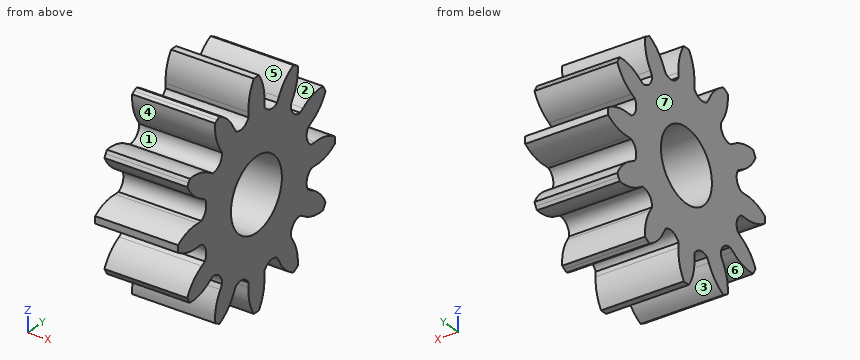
Autodesk Inventor part; units mm, degrees
ref_plane "Work Plane2" through (2.8575, 0, 0) normal (1, 0, 0) x (0, 0, -1)
ref_plane "YZ Plane" through (0, 0, 0) normal (1, 0, 0) x (0, 1, 0)
ref_plane "XZ Plane" through (0, 0, 0) normal (0, 1, 0) x (-1, 0, 0)
ref_plane "Work Plane2" through (2.8575, 0, 0) normal (1, 0, 0) x (0, 0, -1)
sketch "Sketch6" plane through (2.8575, 0, 0) normal (1, 0, 0) x (0, 0, -1)
  line L0 (0.7654, -5.6784) -> (0.7654, -5.022)
  line L1 (-0.7638, -5.6784) -> (-0.7638, -5.0222)
  arc A0 (5.6006, 2.3498) -> (5.5837, 2.3418) centre (6.3532, 0.7382) ccw
  arc A1 (-0.7638, -5.0222) -> (0.7654, -5.022) centre (0, 0) ccw
  line L2 (0.0008, -7.62) -> (-0.2439, -7.62)
  line L3 (0.0008, -7.62) -> (0.2479, -7.62)
  arc A2 (0.2479, -7.62) -> (0.7654, -5.6784) centre (-2.309, -5.8988) ccw
  arc A3 (-0.7638, -5.6784) -> (-0.2439, -7.62) centre (2.2185, -5.9201) ccw
  arc A4 (3.5877, -3.5965) -> (3.5976, -3.5866) centre (0, 0) ccw
  line L4 (3.502, -4.5349) -> (3.1738, -3.9665)
  line L5 (2.1777, -5.2996) -> (1.8496, -4.7313)
  arc A5 (1.8496, -4.7313) -> (3.1738, -3.9665) centre (0, 0) ccw
  line L6 (3.8107, -6.5987) -> (3.5988, -6.721)
  line L7 (3.8107, -6.5987) -> (4.0247, -6.4752)
  arc A6 (4.0247, -6.4752) -> (3.502, -4.5349) centre (0.9498, -6.263) ccw
  arc A7 (2.1777, -5.2996) -> (3.5988, -6.721) centre (4.8813, -4.0177) ccw
  line L8 (5.3003, -2.1764) -> (4.7319, -1.8482)
  line L9 (4.5358, -3.5007) -> (3.9675, -3.1726)
  arc A8 (3.9675, -3.1726) -> (4.7319, -1.8482) centre (0, 0) ccw
  line L10 (6.5995, -3.8093) -> (6.4772, -4.0212)
  line L11 (6.5995, -3.8093) -> (6.7231, -3.5953)
  arc A9 (6.7231, -3.5953) -> (5.3003, -2.1764) centre (3.954, -4.949) ccw
  arc A10 (4.5358, -3.5007) -> (6.4772, -4.0212) centre (6.2362, -1.0388) ccw
  line L12 (5.6784, 0.7654) -> (5.022, 0.7654)
  line L13 (5.6784, -0.7638) -> (5.0222, -0.7638)
  arc A11 (5.0222, -0.7638) -> (5.022, 0.7654) centre (0, 0) ccw
  line L14 (7.62, 0.0008) -> (7.62, -0.2439)
  line L15 (7.62, 0.0008) -> (7.62, 0.2479)
  arc A12 (7.62, 0.2479) -> (5.6784, 0.7654) centre (5.8988, -2.309) ccw
  arc A13 (5.6784, -0.7638) -> (7.62, -0.2439) centre (5.9201, 2.2185) ccw
  line L16 (4.5349, 3.502) -> (3.9665, 3.1738)
  line L17 (5.2996, 2.1777) -> (4.7313, 1.8496)
  arc A14 (4.7313, 1.8496) -> (3.9665, 3.1738) centre (0, 0) ccw
  line L18 (6.5987, 3.8107) -> (6.721, 3.5988)
  line L19 (6.5987, 3.8107) -> (6.4752, 4.0247)
  arc A15 (6.4752, 4.0247) -> (4.5349, 3.502) centre (6.263, 0.9498) ccw
  arc A16 (5.2996, 2.1777) -> (6.721, 3.5988) centre (4.0177, 4.8813) ccw
  line L20 (2.1764, 5.3003) -> (1.8482, 4.7319)
  line L21 (3.5007, 4.5358) -> (3.1726, 3.9675)
  arc A17 (3.1726, 3.9675) -> (1.8482, 4.7319) centre (0, 0) ccw
  line L22 (3.8093, 6.5995) -> (4.0212, 6.4772)
  line L23 (3.8093, 6.5995) -> (3.5953, 6.7231)
  arc A18 (3.5953, 6.7231) -> (2.1764, 5.3003) centre (4.949, 3.954) ccw
  arc A19 (3.5007, 4.5358) -> (4.0212, 6.4772) centre (1.0388, 6.2362) ccw
  line L24 (-0.7654, 5.6784) -> (-0.7654, 5.022)
  line L25 (0.7638, 5.6784) -> (0.7638, 5.0222)
  arc A20 (0.7638, 5.0222) -> (-0.7654, 5.022) centre (0, 0) ccw
  line L26 (-0.0008, 7.62) -> (0.2439, 7.62)
  line L27 (-0.0008, 7.62) -> (-0.2479, 7.62)
  arc A21 (-0.2479, 7.62) -> (-0.7654, 5.6784) centre (2.309, 5.8988) ccw
  arc A22 (0.7638, 5.6784) -> (0.2439, 7.62) centre (-2.2185, 5.9201) ccw
  line L28 (-3.502, 4.5349) -> (-3.1738, 3.9665)
  line L29 (-2.1777, 5.2996) -> (-1.8496, 4.7313)
  arc A23 (-1.8496, 4.7313) -> (-3.1738, 3.9665) centre (0, 0) ccw
  line L30 (-3.8107, 6.5987) -> (-3.5988, 6.721)
  line L31 (-3.8107, 6.5987) -> (-4.0247, 6.4752)
  arc A24 (-4.0247, 6.4752) -> (-3.502, 4.5349) centre (-0.9498, 6.263) ccw
  arc A25 (-2.1777, 5.2996) -> (-3.5988, 6.721) centre (-4.8813, 4.0177) ccw
  line L32 (-5.3003, 2.1764) -> (-4.7319, 1.8482)
  line L33 (-4.5358, 3.5007) -> (-3.9675, 3.1726)
  arc A26 (-3.9675, 3.1726) -> (-4.7319, 1.8482) centre (0, 0) ccw
  line L34 (-6.5995, 3.8093) -> (-6.4772, 4.0212)
  line L35 (-6.5995, 3.8093) -> (-6.7231, 3.5953)
  arc A27 (-6.7231, 3.5953) -> (-5.3003, 2.1764) centre (-3.954, 4.949) ccw
  arc A28 (-4.5358, 3.5007) -> (-6.4772, 4.0212) centre (-6.2362, 1.0388) ccw
  line L36 (-5.6784, -0.7654) -> (-5.022, -0.7654)
  line L37 (-5.6784, 0.7638) -> (-5.0222, 0.7638)
  arc A29 (-5.0222, 0.7638) -> (-5.022, -0.7654) centre (0, 0) ccw
  line L38 (-7.62, -0.0008) -> (-7.62, 0.2439)
  line L39 (-7.62, -0.0008) -> (-7.62, -0.2479)
  arc A30 (-7.62, -0.2479) -> (-5.6784, -0.7654) centre (-5.8988, 2.309) ccw
  arc A31 (-5.6784, 0.7638) -> (-7.62, 0.2439) centre (-5.9201, -2.2185) ccw
  line L40 (-4.5349, -3.502) -> (-3.9665, -3.1738)
  line L41 (-5.2996, -2.1777) -> (-4.7313, -1.8496)
  arc A32 (-4.7313, -1.8496) -> (-3.9665, -3.1738) centre (0, 0) ccw
  line L42 (-6.5987, -3.8107) -> (-6.721, -3.5988)
  line L43 (-6.5987, -3.8107) -> (-6.4752, -4.0247)
  arc A33 (-6.4752, -4.0247) -> (-4.5349, -3.502) centre (-6.263, -0.9498) ccw
  arc A34 (-5.2996, -2.1777) -> (-6.721, -3.5988) centre (-4.0177, -4.8813) ccw
  line L44 (-2.1764, -5.3003) -> (-1.8482, -4.7319)
  line L45 (-3.5007, -4.5358) -> (-3.1726, -3.9675)
  arc A35 (-3.1726, -3.9675) -> (-1.8482, -4.7319) centre (0, 0) ccw
  line L46 (-3.8093, -6.5995) -> (-4.0212, -6.4772)
  line L47 (-3.8093, -6.5995) -> (-3.5953, -6.7231)
  arc A36 (-3.5953, -6.7231) -> (-2.1764, -5.3003) centre (-4.949, -3.954) ccw
  arc A37 (-3.5007, -4.5358) -> (-4.0212, -6.4772) centre (-1.0388, -6.2362) ccw
  arc A38 (-1.8482, -4.7319) -> (-0.7638, -5.0222) centre (0, 0) ccw
  line L48 (-2.0137, 5.0155) -> (-0.7654, 5.3502)
  line L49 (0.7638, 5.3503) -> (2.0123, 5.0161)
  line L50 (3.3367, 4.2516) -> (4.2507, 3.3379)
  line L51 (5.0155, 2.0137) -> (5.3502, 0.7654)
  line L52 (5.3503, -0.7638) -> (5.0161, -2.0123)
  line L53 (4.2516, -3.3367) -> (3.3379, -4.2507)
  line L54 (2.0137, -5.0155) -> (0.7654, -5.3502)
  line L55 (-0.7638, -5.3503) -> (-2.0123, -5.0161)
  line L56 (-3.3367, -4.2516) -> (-4.2507, -3.3379)
  line L57 (-5.0155, -2.0137) -> (-5.3502, -0.7654)
  line L58 (-5.3503, 0.7638) -> (-5.0161, 2.0123)
  line L59 (-4.2516, 3.3367) -> (-3.3379, 4.2507)
  circle A39 centre (0, 0) radius 5.0531
  point P0 (0, 0)
  point P1 (-4.2516, 3.3367)
  dimension "d94" = 360
extrude "Extrusion19" add sketch "Sketch6" against normal blind 5.7277 contours A2 L3 L2 A3 L1 A1 L0 | L0 A1 A38 A35 L45 L56 L40 A32 L41 L57 L36 A29 L37 L58 L32 A26 L33 L59 L28 A23 L29 L48 L24 A20 L25 L49 L20 A17 L21 L50 L16 A14 L17 L51 L12 A11 L13 L52 L8 A8 L9 L53 L4 A5 L5 L54 | L5 A5 L4 A6 L7 L6 A7 | L1 L55 L44 A38 | L44 A36 L47 L46 A37 L45 A35 | L9 A8 L8 A9 L11 L10 A10 | L40 A33 L43 L42 A34 L41 A32 | L13 A11 L12 A12 L15 L14 A13 | L36 A30 L39 L38 A31 L37 A29 | L17 A14 L16 A15 L19 L18 A16 | L32 A27 L35 L34 A28 L33 A26 | L21 A17 L20 A18 L23 L22 A19 | L28 A24 L31 L30 A25 L29 A23 | L25 A20 L24 A21 L27 L26 A22 | A39
sketch "Sketch7" plane through (-2.8702, 0, 0) normal (-1, 0, 0) x (0, 0, 1)
  circle A0 centre (0, 0) radius 2.475
  dimension "d104" = 4.95
extrude "Extrusion20" cut sketch "Sketch7" against normal blind 2540
sketch "Sketch8" plane through (-2.8702, 0, 0) normal (-1, 0, 0) x (0, 0, 1)
  circle A0 centre (0, 0) radius 5.08
  line L0 (-3.3367, 4.2516) -> (-4.2507, 3.3379)
  arc A1 (-4.2507, 3.3379) -> (-3.3367, 4.2516) centre (-4.209, 4.2103) ccw
  line L1 (-3.3367, 4.2516) -> (-3.5007, 4.5358)
  line L2 (-4.2507, 3.3379) -> (-3.3367, 4.2516)
  arc A2 (-5.3502, 0.7654) -> (-5.0155, 2.0137) centre (-5.7503, 1.5417) ccw
  line L3 (-5.3502, 0.7654) -> (-5.0155, 2.0137)
  arc A3 (-5.0161, -2.0123) -> (-5.3503, -0.7638) centre (-5.7507, -1.54) ccw
  line L4 (-5.0161, -2.0123) -> (-5.3503, -0.7638)
  arc A4 (-3.3379, -4.2507) -> (-4.2516, -3.3367) centre (-4.2103, -4.209) ccw
  line L5 (-3.3379, -4.2507) -> (-4.2516, -3.3367)
  arc A5 (-0.7654, -5.3502) -> (-2.0137, -5.0155) centre (-1.5417, -5.7503) ccw
  line L6 (-0.7654, -5.3502) -> (-2.0137, -5.0155)
  arc A6 (2.0123, -5.0161) -> (0.7638, -5.3503) centre (1.54, -5.7507) ccw
  line L7 (2.0123, -5.0161) -> (0.7638, -5.3503)
  arc A7 (4.2507, -3.3379) -> (3.3367, -4.2516) centre (4.209, -4.2103) ccw
  line L8 (4.2507, -3.3379) -> (3.3367, -4.2516)
  arc A8 (5.3502, -0.7654) -> (5.0155, -2.0137) centre (5.7503, -1.5417) ccw
  line L9 (5.3502, -0.7654) -> (5.0155, -2.0137)
  arc A9 (5.0161, 2.0123) -> (5.3503, 0.7638) centre (5.7507, 1.54) ccw
  line L10 (5.0161, 2.0123) -> (5.3503, 0.7638)
  arc A10 (3.3379, 4.2507) -> (4.2516, 3.3367) centre (4.2103, 4.209) ccw
  line L11 (3.3379, 4.2507) -> (4.2516, 3.3367)
  arc A11 (0.7654, 5.3502) -> (2.0137, 5.0155) centre (1.5417, 5.7503) ccw
  line L12 (0.7654, 5.3502) -> (2.0137, 5.0155)
  arc A12 (-2.0123, 5.0161) -> (-0.7638, 5.3503) centre (-1.54, 5.7507) ccw
  line L13 (-2.0123, 5.0161) -> (-0.7638, 5.3503)
  dimension "d107" = 10.16
  dimension "d110" = 360
extrude "Extrusion21" cut sketch "Sketch8" against normal blind 2540 contours A8 L9 | A7 L8 | A6 L7 | A5 L6 | A4 L5 | A3 L4 | A2 L3 | A1 L0 | A12 L13 | A11 L12 | A10 L11 | A9 L10
properties part number "Alligator_Pinion (2)"
Geometry check sheet. Reference: the model listing, model coordinates, mm. Face numbers are marked on the shaded views. A direction names the side the tool comes from. Coordinates: 2 decimals unless noted, no trailing zeros. Write each loop counter-clockwise with the first axis right and the second up, starting at its lowest first coordinate (ties: lowest second). Pieces come first, ordered by that corner, then holes. Notation, with made-up numbers: (-32.75, 4) -> (18.25, 4) arc R26 cw to (18.25, 40) -> close; hole circle Ø4 at (69.25, 42). An arc over 180 degrees is marked (long way). One line per question, with ' | ' between items.
1. Cross-section at C-C on y = -6. Record the cut outline in (x, z).
Answers:
outline: (-2.87, -4.02) -> (2.86, -4.02) -> (2.86, -2.64) -> (-2.87, -2.64) -> close; (-2.87, -0.77) -> (2.86, -0.77) -> (2.86, 0.77) -> (-2.87, 0.77) -> close; (-2.87, 2.64) -> (2.86, 2.64) -> (2.86, 4.02) -> (-2.87, 4.02) -> close
2. Cross-section at A-A on z = 0. Record the cut outline in (x, y) (1 decimal).
Answers:
outline: (-2.9, -7.6) -> (2.9, -7.6) -> (2.9, -2.5) -> (-2.9, -2.5) -> close; (-2.9, 2.5) -> (2.9, 2.5) -> (2.9, 7.6) -> (-2.9, 7.6) -> close
3. Draft check along Y on the marked faces 4, 5, 6 and 7. Enter one of: +Y half, -Y half, draft (parallel to the pull), parting line (faces both ways), or undercut.
Answers:
face 4: -Y half | face 5: undercut | face 6: undercut | face 7: draft
4. Depth check by flat-ended pin: pin 1 Ø2 at (x, z) = (-1, 4.5) entering from -Y; pin 2 Ø1.5 at (x, z) = (-1.5, 5.5) entering from -Y. Enter the tip coordinate at first touch or a pass-through.
Answers:
pin 1: stops at y = -6.72 | pin 2: stops at y = -4.03
5. Cross-section at D-D on z = 3. Record the cut outline in (x, y).
Answers:
outline: (-2.87, -6.34) -> (2.86, -6.34) -> (2.86, 6.34) -> (-2.87, 6.34) -> close
6. Thickness scan on probe 1 along Y at (x, z) = (2.5, 5); probe 2 along Z at (x, y) = (-1, 5.5). Record the ranges inside material, lowest first. Write a range as from..to.
Answers:
probe 1: y = -3.76..-1.99, -1.09..1.09, 1.99..3.76 | probe 2: z = -3.94..-2.28, -0.76..0.77, 2.28..3.94
7. Set-up check for the marked faces 1, 2 and 3: record each of +Z, -Z, +X, -X, +Y, -Y from which the full face is reachable in a straight line by a thin tool's end or side.
Answers:
face 1: +X, -X | face 2: +Z, +X, -X | face 3: -Z, +X, -X
